```python
from build123d import *

# Parameters (mm, degrees)
F0_R     = 38.1
F1_DEPTH = 25.4
F2_R     = 38.1
F3_DEPTH = 38.1
F3_TAPER = 45
F4_R     = 5.08


with BuildPart() as f1:
    # F0 (on Top) → F1 (new body)
    with BuildSketch(Plane.XY):
        Circle(F0_R)
    extrude(amount=F1_DEPTH)

    # F2 (on face) → F3 (join)
    with BuildSketch(Plane.XY.offset(25.4)):
        Circle(F2_R)
    extrude(amount=F3_DEPTH, taper=F3_TAPER)

    # F4
    f4_edges = [f1.edges().sort_by_distance(p)[0] for p in [
        (-38.1, 0, 25.4),
    ]]
    fillet(f4_edges, radius=F4_R)


solid = f1.part
```
Read the model definition and answer for the solid it produces. Units are mm, in the model's axes. Give positions to 0.01 mm unless a question says otherwise; leave off trailing zeros. Write each loop counter-clockwise with the first axis right and the second up, starting at its lowest first coordinate (ties: lowest second). Pieces come first, ordered by that corner, then holes. Notation, with made-up numbers: M 37,12.5 L 52,12.5 A29 ccw 52,40.5 Z; hole C 12,-5.75 d8. An arc over 180 degrees is marked long. Put each result on its own line as item: value. Start each with the question number.
1. Each of these flat-tipped pins is pushed along its axis until it touches: pin 1 Ø12 at (x, z) = (-20, 25.5) entering from -Y; pin 2 Ø6 at (x, z) = (-5.5, 35.5) entering from +Y; pin 3 Ø1.5 at (x, z) = (-19.5, 16) entering from -Y. Where does it stop, or does it pass through?
2. The part is cut by section A-A, the plane z = 12.5. Give the vertices of the cut face in (x, y), and give its area (3 significant figures).
3. Consider line 1 along Z through (x, y) = (18, 17); line 2 along Z through (x, y) = (23.5, -1); line 3 along X through (y, z) = (-9, 46.5). Determine where each line is inside the solid, lowest interval first.
Final values:
1. pin 1: stops at y = -35.31
1. pin 2: stops at y = 30.55
1. pin 3: stops at y = -33.17
2. outline: C 0,0 d76.2
2. area: 4,560 mm²
3. line 1: z = 0 to 38.74
3. line 2: z = 0 to 39.98
3. line 3: x = -14.42 to 14.42
